CAD build for the part. Positions are in the model's coordinates, mm. A direction names the side the tool comes from. Round coordinates to 2 decimals unless told otherwise and drop trailing zeros. Write each loop counter-clockwise with the first axis right and the second up, starting at its lowest first coordinate (ties: lowest second). Pieces come first, ordered by that corner, then holes. Notation, with made-up numbers: (13, 85.5) - (30, 85.5) arc R32 ccw to (30, 114.5) - close; hole circle Ø10 at (70, 7.25). An arc over 180 degrees is marked (long way). Put each result on its own line as item: value. Start each with the question number.
Item 1: Mould opens along Z. For faces 5 (the flat face through (-1, -11, 70)), 6 (the flat face through (-37.32, -2.41, -10.94)), 7 (the flat face through (-1, -11, -70)) say: released by +Z, released by -Z, zero draft, split by the parting line, or undercut.
Item 2: 3-axis set-ups, long thin cutter, end or side, ignore diameter. For faces 1 (the flat face through (-26.847, -2.406, -28.134)), 2 (the flat face through (56, 9.5, -56)), 3 (the cylindrical face through (68.335, 0.133, 15.175)), 4 (the flat face through (-32.819, -5.856, -19.326)): which of +Z, -Z, +X, -X, +Y, -Y reach the whole face in a straight line?
Item 3: Cut at B-B (z = 38). Count the separate pieces of the cut face and the enclosed holes in it, and give its area (3 significant figures).
Item 4: Pin check, flat tips, straight feed: pin 1 Ø7 at (x, z) = (-62.5, -62.5) entering from -Y; pin 2 Ø1 at (y, z) = (-8.5, -6.5) entering from +X; pin 3 Ø16 at (x, z) = (-4, 4.5) entering from -Y; pin 4 Ø3 at (y, z) = (-7, 3) entering from +X. Stop position of each tip, or through.
Item 5: Drill centre lines: line 1 (Y direction, x = -56.5, z = 58.5); line 2 (X direction, y = 1.75, z = 8); line 3 (X direction, y = 1.5, z = -51). Where is each one in solid material? Low to high. Write a range as from..to.
Item 6: Cut at A-A (x = 54). Give the cut face in (y, z), and give its area (3 significant figures).
```python
from build123d import *

# Parameters (mm, degrees)
SKETCH2_OUTSIDE_W         = 258.79
SKETCH2_OUTSIDE_H         = 258.79
SKETCH2_OUTSIDE_W_2       = 140
SKETCH2_OUTSIDE_H_2       = 140
SQUARE_SHAPE_CUTOUT_DEPTH = 144.614066163
MOUNTING_HOLES_START      = -12.5
MOUNTING_HOLES_OUTLINE_R  = 2.25
MOUNTING_HOLES_DEPTH      = 25
FAN_WING_DEPTH            = 2
BOSS_EXTRUDE2_DEPTH       = 5
BOSS_EXTRUDE2_DEPTH_BACK  = 5
SKETCH7_R                 = 10
CIRPATTERN3_COUNT         = 12


# Read off the part's stored shape, not the designer's step: mounting_holes
with BuildPart() as part:
    # Sketch1 → body (revolve)
    with BuildSketch(Plane.XY, mode=Mode.PRIVATE) as body_sk:
        Polygon((67, -12.5), (100, -12.5), (100, -9.5), (70, -9.5), (70, 9.5), (100, 9.5), (100, 12.5), (67, 12.5), align=None)
    revolve(body_sk.sketch.rotate(Axis((0, 0, 0), (0, 1, 0)), 90), axis=Axis((0, 0, 0), (0, 1, 0)))

    # Sketch2 outside → square_shape_cutout (cut, through all)
    with BuildSketch(Plane(origin=(0, 12.5, 0), x_dir=(1, 0, 0), z_dir=(0, 1, 0))):
        Rectangle(SKETCH2_OUTSIDE_W, SKETCH2_OUTSIDE_H)
        Rectangle(SKETCH2_OUTSIDE_W_2, SKETCH2_OUTSIDE_H_2, mode=Mode.SUBTRACT)
    extrude(amount=-SQUARE_SHAPE_CUTOUT_DEPTH, mode=Mode.SUBTRACT)

    # mounting_holes outline → mounting_holes (cut)
    with BuildSketch(Plane(origin=(0, 0, 0), x_dir=(1, 0, 0), z_dir=(0, 1, 0)).offset(MOUNTING_HOLES_START)):
        with Locations((62.5, 62.5)):
            Circle(MOUNTING_HOLES_OUTLINE_R)
        with Locations((-62.5, -62.5)):
            Circle(MOUNTING_HOLES_OUTLINE_R)
        with Locations((62.5, -62.5)):
            Circle(MOUNTING_HOLES_OUTLINE_R)
        with Locations((-62.5, 62.5)):
            Circle(MOUNTING_HOLES_OUTLINE_R)
    extrude(amount=MOUNTING_HOLES_DEPTH, mode=Mode.SUBTRACT)

    # Sketch6 → fan_wing (add)
    with BuildSketch(Plane(origin=(0, 0, 0), x_dir=(0.9433922826162455, -0.3265140162330641, 0.058306074327332945), z_dir=(0.33167906340332987, 0.9287013775293232, -0.16583953170166502))):
        with BuildLine():
            Line((0, 0), (0, 68.153777936))
            ThreePointArc((0, 68.153777936), (-8.870280209, 67.459789157), (-17.540404137, 65.461679426))
            Line((-17.540404137, 65.461679426), (0, 0))
        make_face()
    fan_wing = extrude(amount=FAN_WING_DEPTH)

    # Sketch7 → Boss-Extrude2 (add, two sides: drawn at the far end of the back side and taken through both)
    with BuildSketch(Plane(origin=(0, 0, 0), x_dir=(1, 0, 0), z_dir=(0, 1, 0)).offset(-BOSS_EXTRUDE2_DEPTH_BACK)):
        with Locations(Location((0, 0, 0), (0, 0, 270))):
            Circle(SKETCH7_R)
    extrude(amount=BOSS_EXTRUDE2_DEPTH + BOSS_EXTRUDE2_DEPTH_BACK)

    # CirPattern3: fan_wing ×12 about axis
    cirpattern3_axis = Axis((0, 0, 0), (0, 1, 0))
    for i in range(1, CIRPATTERN3_COUNT):
        add(fan_wing.rotate(cirpattern3_axis, i * 360 / CIRPATTERN3_COUNT))


solid = part.part
```
Output values:
1. face 5: released by +Z
1. face 6: undercut
1. face 7: released by -Z
2. face 1: +Y
2. face 2: -Z, +X
2. face 3: none
2. face 4: -Y
3. separate pieces: 5
3. enclosed holes: 0
3. area: 425 mm2
4. pin 1: y = -12.5
4. pin 2: x = 69.74
4. pin 3: y = -5
4. pin 4: x = 69.98
5. line 1: -12.5..-9.5, 9.5..12.5
5. line 2: -69.54..-66.52, -6..6, 66.52..69.54
5. line 3: -47.95..-43.45, 43.45..47.95
6. outline: (-12.5, -70) - (-9.5, -70) - (-9.5, -44.54) - (9.5, -44.54) - (9.5, -70) - (12.5, -70) - (12.5, -39.66) - (-7.11, -39.66) - (-9.15, -30.41) - (-11.13, -31.18) - (-9.27, -39.66) - (-12.5, -39.66) - close; (-12.5, 39.66) - (12.5, 39.66) - (12.5, 70) - (9.5, 70) - (9.5, 44.54) - (-9.5, 44.54) - (-9.5, 70) - (-12.5, 70) - close; (-11.13, 31.18) - (-4.8, 15.3) - (-2.95, 16.05) - (-9.29, 31.94) - close; (-9.64, 0) - (-4.77, -13.65) - (-2.88, -12.9) - (-7.73, 0.66) - close
6. area: 632 mm2
